Input: part model. Units: mm. Frame: model coordinates. Round coordinates to 2 decimals unless told otherwise and drop trailing zeros. Order: outer loops, then holes, each group sorted by start corner. A loop starts at its lowest first (then second) coordinate and runs counter-clockwise, first axis right, second up. Notation, with made-up numbers: (21.25, 33.5) - (44.25, 33.5) arc R12 cw to (44.25, 39.5) - close; hole circle Ø8 at (69.25, 59). An arc over 180 degrees is marked (long way). One line per item, written item: value. Start each with the question number.
from build123d import *

# Parameters (mm, degrees)
SKETCH4_W           = 320
SKETCH4_H           = 750
BOSS_EXTRUDE3_DEPTH = 8
CUT_EXTRUDE1_DEPTH  = 8


with BuildPart() as part:
    # Sketch4 → Boss-Extrude3 (new body)
    with BuildSketch(Plane(origin=(0, 0, 0), x_dir=(1, 0, 0), z_dir=(0, 1, 0))):
        with Locations((160, 375)):
            Rectangle(SKETCH4_W, SKETCH4_H)
    extrude(amount=BOSS_EXTRUDE3_DEPTH)

    # Sketch8 → Cut-Extrude1 (cut)
    with BuildSketch(Plane(origin=(0, 8, 0), x_dir=(1, 0, 0), z_dir=(0, 1, 0))):
        with BuildLine():
            Line((119, 100), (58, 100))
            ThreePointArc((58, 100), (54.464466094, 101.464466094), (53, 105))
            Line((53, 105), (53, 268.675816019))
            ThreePointArc((53, 268.675816019), (54.464466094, 272.211349925), (58, 273.675816019))
            Line((58, 273.675816019), (119, 273.675816019))
            ThreePointArc((119, 273.675816019), (122.535533906, 272.211349925), (124, 268.675816019))
            Line((124, 268.675816019), (124, 105))
            ThreePointArc((124, 105), (122.535533906, 101.464466094), (119, 100))
        make_face()
        with BuildLine():
            Line((230, 225), (230, 525))
            ThreePointArc((230, 525), (255, 550), (280, 525))
            Line((280, 525), (280, 225))
            ThreePointArc((280, 225), (255, 200), (230, 225))
        make_face()
        with BuildLine():
            Line((119, 476.324183981), (58, 476.324183981))
            ThreePointArc((58, 476.324183981), (54.464466094, 477.788650075), (53, 481.324183981))
            Line((53, 481.324183981), (53, 645))
            ThreePointArc((53, 645), (54.464466094, 648.535533906), (58, 650))
            Line((58, 650), (119, 650))
            ThreePointArc((119, 650), (122.535533906, 648.535533906), (124, 645))
            Line((124, 645), (124, 481.324183981))
            ThreePointArc((124, 481.324183981), (122.535533906, 477.788650075), (119, 476.324183981))
        make_face()
    extrude(amount=-CUT_EXTRUDE1_DEPTH, mode=Mode.SUBTRACT)


solid = part.part
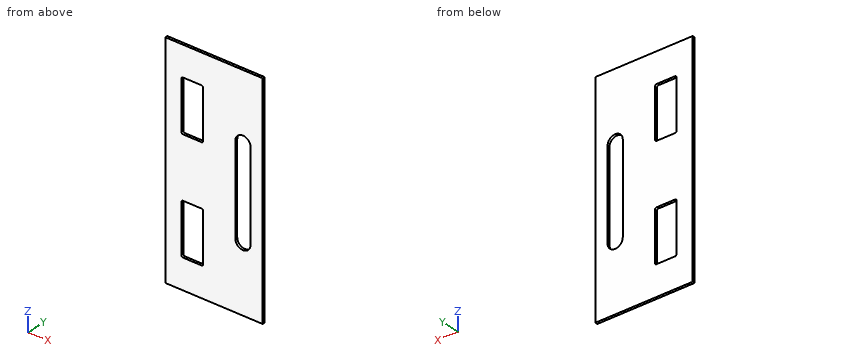
Item 1: Section query D-D on y = 3.25. Return loops of the section in (x, z).
Item 2: Line query: L1, parallel to X at y = 2, z = -495.5; L2, parallel to Z at x = 115, y = 1.25; L3, parallel to X at y = 2.5, z = -168. Output: solid intervals per line, ascending.
Item 3: Section query A-A on z = -499.5. Return loops of the section in (x, y).
Item 4: Section query B-B on x = 255. Return loops of the section in (y, z).
Item 5: Section query C-C on x = 103. Return loops of the section in (y, z), and give its area (3 significant figures).
Item 6: First-contact query: pin 1 Ø1.5 at (x, y) = (32, 4) entering from +Z. Flat tip, straight axial feed; report the tip coordinate or a pass-through.
Geometry results:
1. outline: (0, -750) - (320, -750) - (320, 0) - (0, 0) - close; hole (53, -645) arc R5 ccw to (58, -650) - (119, -650) arc R5 ccw to (124, -645) - (124, -481.32) arc R5 ccw to (119, -476.32) - (58, -476.32) arc R5 ccw to (53, -481.32) - close; hole (53, -268.68) arc R5 ccw to (58, -273.68) - (119, -273.68) arc R5 ccw to (124, -268.68) - (124, -105) arc R5 ccw to (119, -100) - (58, -100) arc R5 ccw to (53, -105) - close; hole (230, -525) arc R25 ccw to (280, -525) - (280, -225) arc R25 ccw to (230, -225) - close
2. L1: x = 0 to 53, 124 to 230, 280 to 320
2. L2: z = -750 to -650, -476.32 to -273.68, -100 to 0
2. L3: x = 0 to 53, 124 to 320
3. outline: (0, 0) - (53, 0) - (53, 8) - (0, 8) - close; (124, 0) - (230, 0) - (230, 8) - (124, 8) - close; (280, 0) - (320, 0) - (320, 8) - (280, 8) - close
4. outline: (0, -750) - (8, -750) - (8, -550) - (0, -550) - close; (0, -200) - (8, -200) - (8, 0) - (0, 0) - close
5. outline: (0, -750) - (8, -750) - (8, -650) - (0, -650) - close; (0, -476.32) - (8, -476.32) - (8, -273.68) - (0, -273.68) - close; (0, -100) - (8, -100) - (8, 0) - (0, 0) - close
5. area: 3,220 mm^2
6. pin 1: stops at z = 0
